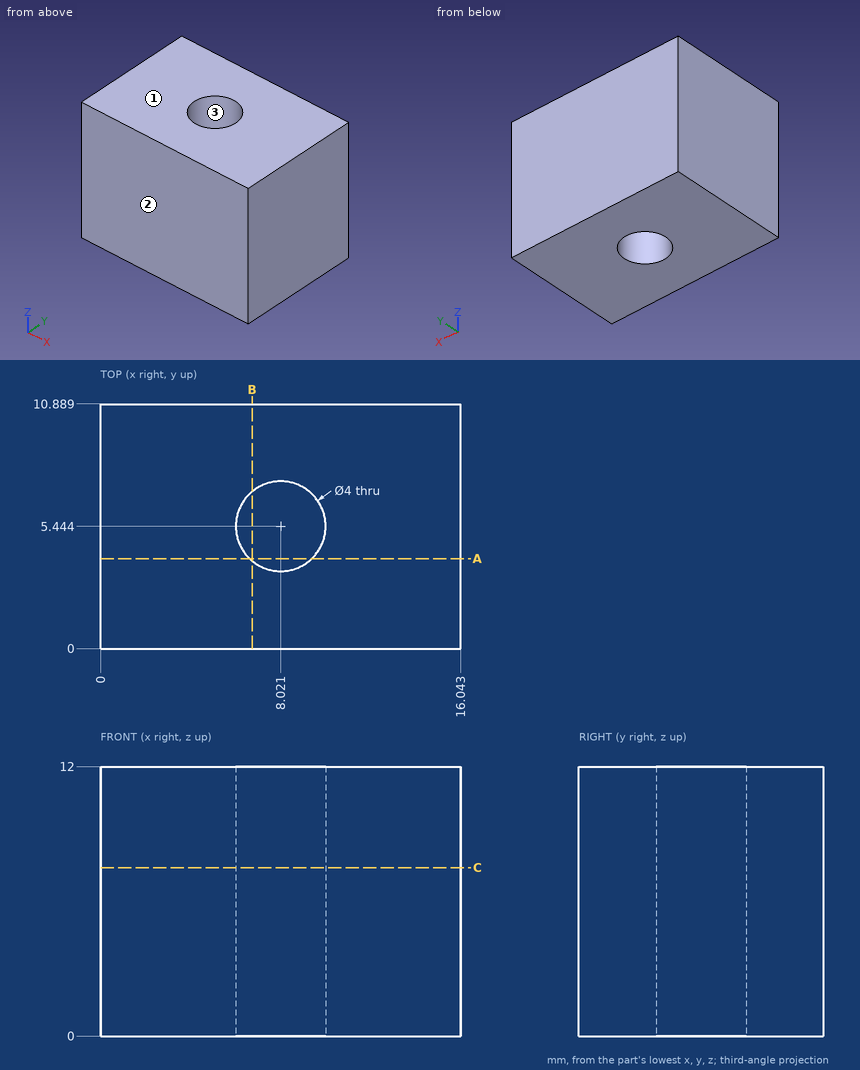
Design review of the part shown in the three views and the two pictorial views. Dimensions are in mm from the part's minimum x, y and z. Give positions to 0.01 mm unless a question says otherwise; leave off trailing zeros. Write each loop counter-clockwise with the first axis right and the second up, starting at its lowest first coordinate (ties: lowest second). Pieces come first, ordered by that corner, then holes. Notation, with made-up numbers: M 69.5,43 L 82.5,43 A19 ccw 82.5,55 Z; hole C -23,-4 d6. An arc over 180 degrees is marked long. Return JSON: item names as keys, results as strings. Group by question number.
Item 1: Take a section at A-A (y = 4). Give the boundary of the cut face in (x, z) (1 decimal), plus the area to 3 significant figures.
Item 2: Wall thickness on line 1 along X through (y, z) = (4, 10.5) (1 decimal); line 2 along X through (y, z) = (4.75, 7.5) (1 decimal): over which ranges is each line inside the solid? List them lowest first.
Item 3: Take a section at B-B (x = 6.75). Give the boundary of the cut face in (y, z).
Item 4: Take a section at C-C (z = 7.5). Give the boundary of the cut face in (x, y) (1 decimal).
Item 5: The part is to be moulded in two halves that separate along Y. For the marked faces 1, 2 and 3, say which applies: pulls with the +Y half, pulls with the -Y half, needs draft (parallel to the pull), parting line crosses it, or undercut.
Item 6: Clearance check with a flat-ended pin moving along its axis: pin 1 Ø3.5 at (x, y) = (8.02, 5.44) entering from +Z. State where the tip first meets the part, or that it passes through.
Return value:
{
 "1": {"outline": "M 0,0 L 6.6,0 L 6.6,12 L 0,12 Z; M 9.4,0 L 16,0 L 16,12 L 9.4,12 Z", "area": "159 mm2"},
 "2": {"line 1": "x = 0 to 6.6, 9.4 to 16", "line 2": "x = 0 to 6.1, 9.9 to 16"},
 "3": {"outline": "M 0,0 L 3.9,0 L 3.9,12 L 0,12 Z; M 6.99,0 L 10.89,0 L 10.89,12 L 6.99,12 Z"},
 "4": {"outline": "M 0,0 L 16,0 L 16,10.9 L 0,10.9 Z; hole C 8,5.4 d4"},
 "5": {"face 1": "needs draft", "face 2": "pulls with the -Y half", "face 3": "undercut"},
 "6": {"pin 1": "passes through"}
}
